Part model, mm, in its own coordinate system. Face numbers are marked on the shaded views. A direction names the side the tool comes from. Round coordinates to 2 decimals unless told otherwise and drop trailing zeros. Write each loop counter-clockwise with the first axis right and the second up, starting at its lowest first coordinate (ties: lowest second). Pieces come first, ordered by that corner, then holes. Notation, with made-up numbers: (36.25, -20) -> (80.25, -20) arc R15 ccw to (80.25, -9) -> close; hole circle Ø11 at (-16, -39.75). An arc over 180 degrees is marked (long way). Return JSON: item names as keys, results as strings. Group by question number.
(1) Saw through at C-C (z = 8). List the corners of the cut face in (x, y).
(2) Saw through at A-A (y = 6). List the corners of the cut face in (x, z).
(3) Mould opens along Z. For the marked faces 3, 4 and 5 say: +Z half, -Z half, draft (parallel to the pull), parting line (faces both ways), or undercut.
(4) Tool access for the marked faces 1 and 2: list every direction of +Z, -Z, +X, -X, +Y, -Y with a clear straight run to the whole face (end or side of a thin tool).
(5) Drop a flat-ended pin along its axis: pin 1 Ø10.5 at (x, z) = (8, 13.5) entering from +Y. Give the stop position or say it passes through.
(6) Saw through at B-B (x = 9.5). List the corners of the cut face in (y, z).
(7) Drill centre lines: L1, parallel to Z at x = -5.5, y = 4.5; L2, parallel to Y at x = -13, z = -36.5; L3, parallel to Y at x = -9.5, z = 40.05. Where is each one in solid material? Low to high. Write a range as from..to.
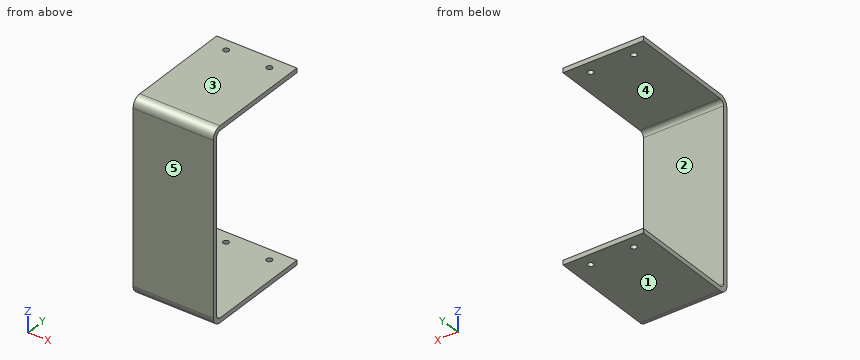
from build123d import *

# Parameters (mm, degrees)
SKETCH1_W                      = 35
SKETCH1_H                      = 83
BASE_FLANGE2_DEPTH             = 2
EDGE_FLANGE3_STRIP_W           = 12
EDGE_FLANGE3_STRIP_H           = 2
EDGE_FLANGE3_STRIP_CUT_DEPTH   = 35
EDGE_FLANGE3_STRIP_2_W         = 12
EDGE_FLANGE3_STRIP_2_H         = 2
EDGE_FLANGE3_STRIP_CUT_2_DEPTH = 35
EDGE_FLANGE3_DEPTH             = 35
EDGE_FLANGE3_BEND_DEPTH        = 35
TAP_DRILL_FOR_M3_TAP1_D        = 2.5


# Sheet-metal steps are written as plain solids
with BuildPart() as part:
    # Sketch1 → Base-Flange2 (new body)
    with BuildSketch(Plane(origin=(0, 0, 0), x_dir=(1, 0, 0), z_dir=(0, 1, 0))):
        Rectangle(SKETCH1_W, SKETCH1_H)
    extrude(amount=-BASE_FLANGE2_DEPTH)

    # Edge-Flange3 strip (across the edge) → Edge-Flange3 strip cut (cut)
    with BuildSketch(Plane(origin=(17.5, 0, -41.5), x_dir=(0, 0, 1), z_dir=(-1, 0, 0))):
        with Locations((-2, -1)):
            Rectangle(EDGE_FLANGE3_STRIP_W, EDGE_FLANGE3_STRIP_H)
    extrude(amount=EDGE_FLANGE3_STRIP_CUT_DEPTH, mode=Mode.SUBTRACT)

    # Edge-Flange3 strip 2 (across the edge) → Edge-Flange3 strip cut 2 (cut)
    with BuildSketch(Plane(origin=(-17.5, 0, 41.5), x_dir=(0, 0, -1), z_dir=(1, 0, 0))):
        with Locations((-2, -1)):
            Rectangle(EDGE_FLANGE3_STRIP_2_W, EDGE_FLANGE3_STRIP_2_H)
    extrude(amount=EDGE_FLANGE3_STRIP_CUT_2_DEPTH, mode=Mode.SUBTRACT)

    # Edge-Flange3 section (across the edge) → Edge-Flange3 (add)
    with BuildSketch(Plane(origin=(17.5, 0, -41.5), x_dir=(0, 0, 1), z_dir=(-1, 0, 0))):
        with BuildLine():
            Line((0, 2), (0, 48))
            Line((0, 48), (2, 48))
            Line((2, 48), (2, 2))
            ThreePointArc((2, 2), (2.585786438, 0.585786438), (4, 0))
            Line((4, 0), (4, -2))
            ThreePointArc((4, -2), (1.171572875, -0.828427125), (0, 2))
        make_face()
    extrude(amount=EDGE_FLANGE3_DEPTH)

    # Edge-Flange3 section 2 (across the edge) → Edge-Flange3 bend (add)
    with BuildSketch(Plane(origin=(-17.5, 0, 41.5), x_dir=(0, 0, -1), z_dir=(1, 0, 0))):
        with BuildLine():
            Line((0, 2), (0, 48))
            Line((0, 48), (2, 48))
            Line((2, 48), (2, 2))
            ThreePointArc((2, 2), (2.585786438, 0.585786438), (4, 0))
            Line((4, 0), (4, -2))
            ThreePointArc((4, -2), (1.171572875, -0.828427125), (0, 2))
        make_face()
    extrude(amount=EDGE_FLANGE3_BEND_DEPTH)

    # Tap Drill for M3 Tap1 (through all)
    with Locations(Plane(origin=(-15.830402425, -23.069767603, -43.5), x_dir=(-1, 0, 0), z_dir=(0, 0, -1))):
        with Locations((-25.330402425, 65.569767603), (-6.330402425, 65.739876607)):
            Hole(TAP_DRILL_FOR_M3_TAP1_D / 2)


solid = part.part
Computed values:
{
 "1": {"outline": "(-17.5, -2) -> (17.5, -2) -> (17.5, 0) -> (-17.5, 0) -> close"},
 "2": {"outline": "(-17.5, -41.5) -> (17.5, -41.5) -> (17.5, -39.5) -> (-17.5, -39.5) -> close; (-17.5, 39.5) -> (17.5, 39.5) -> (17.5, 41.5) -> (-17.5, 41.5) -> close"},
 "3": {"face 3": "+Z half", "face 4": "undercut", "face 5": "draft"},
 "4": {"face 1": "-Z, +X, -X, +Y, -Y", "face 2": "+X, -X, +Y"},
 "5": {"pin 1": "y = 0"},
 "6": {"outline": "(-2, -37.5) arc R4 ccw to (2, -41.5) -> (41.25, -41.5) -> (41.25, -39.5) -> (2, -39.5) arc R2 cw to (0, -37.5) -> (0, 37.5) arc R2 cw to (2, 39.5) -> (41.25, 39.5) -> (41.25, 41.5) -> (2, 41.5) arc R4 ccw to (-2, 37.5) -> close; (43.75, -41.5) -> (48, -41.5) -> (48, -39.5) -> (43.75, -39.5) -> close; (43.75, 39.5) -> (48, 39.5) -> (48, 41.5) -> (43.75, 41.5) -> close"},
 "7": {"L1": "-41.5..-39.5, 39.5..41.5", "L2": "-2..0", "L3": "-1.08..41.42, 43.92..48"}
}
